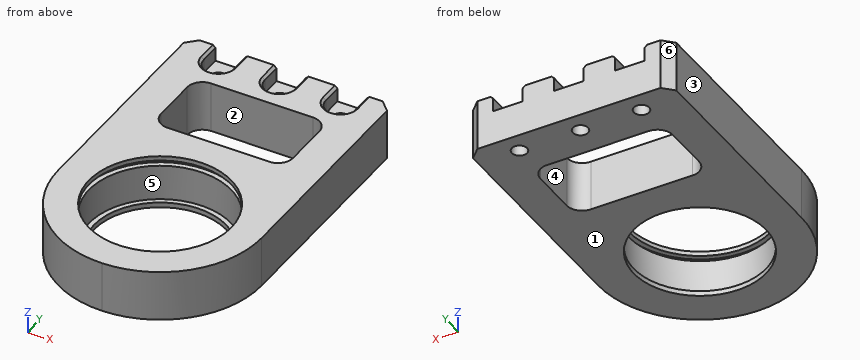
```python
from build123d import *

# Parameters (mm, degrees)
SKETCH_1_W          = 40
SKETCH_1_H          = 65
EXTRUDE_1_DEPTH     = 10
SKETCH_2_R          = 14
CUT_EXTRUDE_1_DEPTH = 12
SKETCH_3_R          = 15.05
CUT_EXTRUDE_2_DEPTH = 1.1
CHAMFER_1_SIZE      = 2
FILLET_1_R          = 20
SKETCH_4_R          = 1.5
CUT_EXTRUDE_3_DEPTH = 15
SKETCH_5_W          = 26
SKETCH_5_H          = 15
CUT_EXTRUDE_4_DEPTH = 15
FILLET_2_R          = 3
EXTRUDE_START       = -1
SKETCH_7_R          = 14
SKETCH_7_R_2        = 13
EXTRUDE_2_DEPTH     = 1
CUT_EXTRUDE_5_DEPTH = 3.2
CHAMFER_2_SIZE      = 0.5


with BuildPart() as part:
    # 草图1 → 凸台-拉伸1 (new body)
    with BuildSketch(Plane.XY):
        with Locations((20, -37.5)):
            Rectangle(SKETCH_1_W, SKETCH_1_H)
    extrude(amount=EXTRUDE_1_DEPTH)

    # 草图2 → 切除-拉伸1 (cut)
    with BuildSketch(Plane.XY.offset(10)):
        with Locations((20, -50)):
            Circle(SKETCH_2_R)
    extrude(amount=-CUT_EXTRUDE_1_DEPTH, mode=Mode.SUBTRACT)

    # 草图3 → 切除-拉伸2 (cut)
    with BuildSketch(Plane(origin=(0, 0, 8), x_dir=(-1, 0, 0), z_dir=(0, 0, -1))):
        with Locations((-20, -50)):
            Circle(SKETCH_3_R)
    extrude(amount=-CUT_EXTRUDE_2_DEPTH, mode=Mode.SUBTRACT)

    # 倒角1
    chamfer_1_edges = [part.edges().sort_by_distance(p)[0] for p in [
        (0, -5, 5),
        (40, -5, 5),
    ]]
    chamfer(chamfer_1_edges, length=CHAMFER_1_SIZE)

    # 圆角1
    fillet_1_edges = [part.edges().sort_by_distance(p)[0] for p in [
        (0, -70, 5),
        (40, -70, 5),
    ]]
    fillet(fillet_1_edges, radius=FILLET_1_R - 0.0001)  # a hair under: the kernel refuses the full size

    # 草图4 → 切除-拉伸3 (cut)
    with BuildSketch(Plane(origin=(0, 0, 0), x_dir=(-1, 0, 0), z_dir=(0, 0, -1))):
        with Locations((-32, -9)):
            Circle(SKETCH_4_R)
        with Locations((-20, -9)):
            Circle(SKETCH_4_R)
        with Locations((-8, -9)):
            Circle(SKETCH_4_R)
    extrude(amount=-CUT_EXTRUDE_3_DEPTH, mode=Mode.SUBTRACT)

    # 草图5 → 切除-拉伸4 (cut)
    with BuildSketch(Plane(origin=(0, 0, 0), x_dir=(-1, 0, 0), z_dir=(0, 0, -1))):
        with Locations((-20, -22.5)):
            Rectangle(SKETCH_5_W, SKETCH_5_H)
    extrude(amount=-CUT_EXTRUDE_4_DEPTH, mode=Mode.SUBTRACT)

    # 圆角2
    fillet_2_edges = [part.edges().sort_by_distance(p)[0] for p in [
        (7, -15, 5),
        (7, -30, 5),
        (33, -30, 5),
        (33, -15, 5),
    ]]
    fillet(fillet_2_edges, radius=FILLET_2_R)

    # 草图7 → 凸台-拉伸2 (add)
    with BuildSketch(Plane(origin=(0, 0, 0), x_dir=(-1, 0, 0), z_dir=(0, 0, -1)).offset(EXTRUDE_START)):
        with Locations((-20, -50)):
            Circle(SKETCH_7_R)
        with Locations((-20, -50)):
            Circle(SKETCH_7_R_2, mode=Mode.SUBTRACT)
    extrude(amount=EXTRUDE_2_DEPTH)

    # 草图8 → 切除-拉伸5 (cut)
    with BuildSketch(Plane.XY.offset(10)):
        with BuildLine():
            Line((5.1, -9), (5.1, -5))
            Line((5.1, -5), (10.9, -5))
            Line((10.9, -5), (10.9, -9))
            ThreePointArc((10.9, -9), (8, -11.9), (5.1, -9))
        make_face()
        with BuildLine():
            Line((17.1, -9), (17.1, -5))
            Line((17.1, -5), (22.9, -5))
            Line((22.9, -5), (22.9, -9))
            ThreePointArc((22.9, -9), (20, -11.9), (17.1, -9))
        make_face()
        with BuildLine():
            Line((34.9, -9), (34.9, -5))
            Line((34.9, -5), (29.1, -5))
            Line((29.1, -5), (29.1, -9))
            ThreePointArc((29.1, -9), (32, -11.9), (34.9, -9))
        make_face()
    extrude(amount=-CUT_EXTRUDE_5_DEPTH, mode=Mode.SUBTRACT)

    # 倒角2
    chamfer_2_edges = [part.edges().sort_by_distance(p)[0] for p in [
        (8, -11.9, 10),
        (10.9, -7, 10),
        (5.1, -7, 10),
        (32, -11.9, 10),
        (34.9, -7, 10),
        (29.1, -7, 10),
        (20, -11.9, 10),
        (22.9, -7, 10),
        (17.1, -7, 10),
    ]]
    chamfer(chamfer_2_edges, length=CHAMFER_2_SIZE)


solid = part.part
```
The model under review builds one solid part; all positions refer to its coordinate system, in mm. Face numbers are marked on the shaded views. A direction names the side the tool comes from. Round coordinates to 2 decimals unless told otherwise and drop trailing zeros. Write each loop counter-clockwise with the first axis right and the second up, starting at its lowest first coordinate (ties: lowest second). Pieces come first, ordered by that corner, then holes. Notation, with made-up numbers: (-32, 9.5) - (19, 9.5) arc R27 ccw to (19, 28.5) - close; hole circle Ø6 at (84.25, 12.5). An arc over 180 degrees is marked (long way). One line per question, with ' | ' between items.
Item 1: To check wall thickness, follow probe 1 along Y at (x, z) = (20, 4.5); probe 2 along Y at (x, z) = (20, 8.45); probe 3 along X at (y, z) = (-8.5, 7.75). State the ranges of each line that lie inside material, in increasing order.
Resolved:
probe 1: y = -70 to -64, -36 to -30, -15 to -10.5, -7.5 to -5 | probe 2: y = -70 to -65.05, -34.95 to -30, -15 to -11.9 | probe 3: x = 0 to 5.1, 10.9 to 17.1, 22.9 to 29.1, 34.9 to 40
Item 2: Add section A-A, the plane y = -23. Give the boundary of the cut face in (x, z).
Resolved:
outline: (0, 0) - (7, 0) - (7, 10) - (0, 10) - close; (33, 0) - (40, 0) - (40, 10) - (33, 10) - close
Item 3: For P1, Ø14, axis at x = 17, y = -50.5, coming from the +Z side; P2, Ø6, axis at x = 23.5, z = 4, coming from the -Y side; P3, Ø3, axis at x = 23.5, z = 7, coming from the -Y side, all flat-tipped, find the tip position at first contact; note any pin that passes through.
Resolved:
P1: passes through | P2: stops at y = -69.99 | P3: stops at y = -69.9
Item 4: For the marked faces 4, 5 and 6, list the 3-axis set-ups (+Z, -Z, +X, -X, +Y, -Y) from which the entire face can be reached by the end or side of a thin tool; tool diameter is ignored.
Resolved:
face 4: +Z, -Z | face 5: +Z | face 6: +Z, -Z, -X, +Y
Item 5: Add section D-D, the plane y = -40. Give the boundary of the cut face in (x, z).
Resolved:
outline: (0, 0) - (11.69, 0) - (11.69, 1) - (10.2, 1) - (10.2, 8) - (8.75, 8) - (8.75, 9.1) - (10.2, 9.1) - (10.2, 10) - (0, 10) - close; (28.31, 0) - (40, 0) - (40, 10) - (29.8, 10) - (29.8, 9.1) - (31.25, 9.1) - (31.25, 8) - (29.8, 8) - (29.8, 1) - (28.31, 1) - close
Item 6: Add section B-B, the plane x = 14. Give the boundary of the cut face in (y, z), then the cut area to 3 significant figures.
Resolved:
outline: (-69.08, 0) - (-61.53, 0) - (-61.53, 1) - (-62.65, 1) - (-62.65, 8) - (-63.8, 8) - (-63.8, 9.1) - (-62.65, 9.1) - (-62.65, 10) - (-69.08, 10) - close; (-38.47, 0) - (-30, 0) - (-30, 10) - (-37.35, 10) - (-37.35, 9.1) - (-36.2, 9.1) - (-36.2, 8) - (-37.35, 8) - (-37.35, 1) - (-38.47, 1) - close; (-15, 0) - (-5, 0) - (-5, 10) - (-15, 10) - close | area: 238 mm2
Item 7: Add section C-C, the plane x = 8. State how many separate pieces and enclosed holes the cut face has, then the cut area to 3 significant figures.
Resolved:
separate pieces: 4 | enclosed holes: 0 | area: 289 mm2
Item 8: The part is to be moulded in two halves that separate along X. For the marked faces 1, 2 and 3, say which applies: pulls with the +X half, pulls with the -X half, needs draft (parallel to the pull), parting line crosses it, or undercut.
Resolved:
face 1: needs draft | face 2: undercut | face 3: pulls with the -X half
